Autodesk Inventor part; units mm, degrees
ref_plane "YZ Plane" through (0, 0, 0) normal (1, 0, 0) x (0, 1, 0)
ref_plane "XZ Plane" through (0, 0, 0) normal (0, 1, 0) x (-1, 0, 0)
ref_plane "XY Plane" through (0, 0, 0) normal (0, 0, 1) x (1, 0, 0)
sketch "Block1" plane through (0, 0, 0) normal (0, 0, 1) x (1, 0, 0)
  line L0 (-60.22, 0.22) -> (-60.22, -150.22)
  line L1 (-60.22, -150.22) -> (0.22, -150.22)
  line L2 (0.22, -150.22) -> (0.22, 0.22)
  line L3 (0.22, 0.22) -> (-60.22, 0.22)
  circle A0 centre (-30, -20) radius 5.22
  circle A1 centre (-30, -130) radius 5.22
  point P0 (-30, -75)
sketch "Sketch1" plane through (0, 0, 0) normal (0, 1, 0) x (-1, 0, 0)
  line L0 (0, 0) -> (60, 0)
  line L1 (60, 0) -> (60, 150)
  line L2 (60, 150) -> (0, 150)
  line L3 (0, 150) -> (0, 0)
  circle A0 centre (30, 130) radius 5
  circle A1 centre (30, 20) radius 5
  dimension "d0" = 60
  dimension "d1" = 150
  dimension "d4" = 10
  dimension "d5" = 10
  dimension "d6" = 20
  dimension "d7" = 20
  dimension "d8" = 30
  dimension "d11" = 30
extrude "Extrusion2" add sketch "Sketch1" along normal blind 20
sketch "Sketch2" plane through (0, 20, 0) normal (0, 1, 0) x (1, 0, 0)
  line L0 (0, -150) -> (0, 0)
  line L1 (-60, -150) -> (0, -150)
  line L2 (-60, 0) -> (-60, -150)
  circle A0 centre (-30, -130) radius 5
  circle A1 centre (-30, -20) radius 5
  line L3 (0, 0) -> (-60, 0)
sketch "DXF" plane through (0, 0, 0) normal (0, 1, 0) x (-1, 0, 0)
  point P0 (0, 0)
equation "\"d8\" = 0.5 * d0"
equation "\"d11\" = 0.5 * d0"
properties part number "holderBlock"
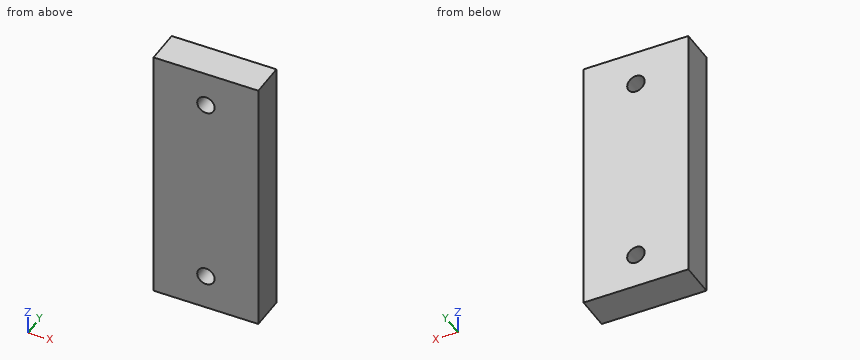
Model file for the job. Use its own axes, mm. Give positions to 0.01 mm unless a question says otherwise; leave off trailing zeros. Write each loop counter-clockwise with the first axis right and the second up, starting at its lowest first coordinate (ties: lowest second). Pieces come first, ordered by that corner, then holes. Notation, with made-up numbers: (30, 45) -> (39, 45) arc R4 ccw to (39, 50) -> close; hole circle Ø10 at (87, 83.5). An arc over 180 degrees is marked (long way). Use CSV: the item, a comma, the result in double quotes. Start each with the question number.
1) Cut at B-B on x = -30. List the corners of the cut face in (y, z).
2) Cut at A-A on z = 130. List the corners of the cut face in (x, y), plus the area to 3 significant figures.
3) Drill centre lines: L1, parallel to Z at x = -30, y = 9; L2, parallel to Z at x = -32.5, y = 9; L3, parallel to X at y = 2.5, z = 131.5. Where is each one in solid material? Low to high.
4) Cut at C-C on y = 7.5. List the corners of the cut face in (x, z), plus the area to 3 significant figures.
5) Pin check, flat tip, straight feed: P1, Ø2, axis at x = -47.5, z = 95, coming from the -Y side. Stop position of the tip, or through.
Final values:
1,outline,"(0, 0) -> (20, 0) -> (20, 15) -> (0, 15) -> close; (0, 25) -> (20, 25) -> (20, 125) -> (0, 125) -> close; (0, 135) -> (20, 135) -> (20, 150) -> (0, 150) -> close"
2,outline,"(-60, 0) -> (-35, 0) -> (-35, 20) -> (-60, 20) -> close; (-25, 0) -> (0, 0) -> (0, 20) -> (-25, 20) -> close"
2,area,"1,000 mm2"
3,L1,"z = 0 to 15, 25 to 125, 135 to 150"
3,L2,"z = 0 to 15.67, 24.33 to 125.67, 134.33 to 150"
3,L3,"x = -60 to -34.77, -25.23 to 0"
4,outline,"(-60, 0) -> (0, 0) -> (0, 150) -> (-60, 150) -> close; hole circle Ø10 at (-30, 20); hole circle Ø10 at (-30, 130)"
4,area,"8,840 mm2"
5,P1,"stops at y = 0"
